Part model, mm, in its own coordinate system. A direction names the side the tool comes from. Give positions to 0.01 mm unless a question says otherwise; leave off trailing zeros. Loops run counter-clockwise (first coordinate to the right, second up) from the corner with the lowest first, then second, coordinate; pieces in that order, holes last. Notation, with made-up numbers: M 58.5,80 L 100.5,80 A31 cw 100.5,108 Z; hole C -36.5,37.25 d9. An arc over 180 degrees is marked long. Answer in a Markdown table with one row per item.
from build123d import *

# Parameters (mm, degrees)
SKETCH1_W                       = 101.6
SKETCH1_H                       = 59.436
BASE_EXTRUDE_DEPTH              = 3.81
BASE_CORNER_FILLET_R            = 2.54
SKETCH3_W                       = 3.81
SKETCH3_H                       = 3.81
PEG_EXTRUDE_DEPTH               = 2.54
MATERIAL_REMOVAL_CUT_DEPTH      = 120.96788652
SKETCH5_R                       = 1.905
REMOTE_CONTROL_HOLDER_CUT_DEPTH = 120.96788652


with BuildPart() as part:
    # Sketch1 → Base Extrude (new body)
    with BuildSketch(Plane(origin=(0, 0, 0), x_dir=(1, 0, 0), z_dir=(0, 1, 0))):
        with Locations((50.8, 29.718)):
            Rectangle(SKETCH1_W, SKETCH1_H)
    extrude(amount=BASE_EXTRUDE_DEPTH)

    # Base Corner Fillet
    base_corner_fillet_edges = [part.edges().sort_by_distance(p)[0] for p in [
        (0, 1.905, -59.436),
        (101.6, 1.905, -59.436),
        (101.6, 1.905, 0),
        (0, 1.905, 0),
    ]]
    fillet(base_corner_fillet_edges, radius=BASE_CORNER_FILLET_R)

    # Sketch3 → Peg Extrude (add)
    with BuildSketch(Plane.ZY):
        with Locations((-20.193, 1.905)):
            Rectangle(SKETCH3_W, SKETCH3_H)
        with Locations((-39.243, 1.905)):
            Rectangle(SKETCH3_W, SKETCH3_H)
    peg_extrude = extrude(amount=PEG_EXTRUDE_DEPTH)

    # Peg Mirror: Peg Extrude across plane
    add(peg_extrude.mirror(Plane(origin=(50.8, 0, 0), x_dir=(0, 0, 1), z_dir=(1, 0, 0))))

    # Sketch4 → Material Removal Cut (cut, through all)
    with BuildSketch(Plane.XZ):
        with BuildLine():
            Line((19.05, -12.7), (82.55, -12.7))
            ThreePointArc((82.55, -12.7), (87.040128061, -14.559871939), (88.9, -19.05))
            Line((88.9, -19.05), (88.9, -40.386))
            ThreePointArc((88.9, -40.386), (87.040128061, -44.876128061), (82.55, -46.736))
            Line((82.55, -46.736), (19.05, -46.736))
            ThreePointArc((19.05, -46.736), (14.559871939, -44.876128061), (12.7, -40.386))
            Line((12.7, -40.386), (12.7, -19.05))
            ThreePointArc((12.7, -19.05), (14.559871939, -14.559871939), (19.05, -12.7))
        make_face()
    extrude(amount=-MATERIAL_REMOVAL_CUT_DEPTH, mode=Mode.SUBTRACT)

    # Sketch5 → Remote Control Holder Cut (cut, through all)
    with BuildSketch(Plane(origin=(0, 3.81, 0), x_dir=(1, 0, 0), z_dir=(0, 1, 0))):
        with Locations(Location((63.5, 4.318, 0), (0, 0, 270))):
            Circle(SKETCH5_R)
        with Locations(Location((63.5, 55.118, 0), (0, 0, 270))):
            Circle(SKETCH5_R)
    extrude(amount=-REMOTE_CONTROL_HOLDER_CUT_DEPTH, mode=Mode.SUBTRACT)


solid = part.part
(1) Saw through at A-A (z = -32). Write the cut outline in (x, y), plus the area to 3 significant figures.
Recorded:
| item | result |
|---|---|
| outline | M 0,0 L 12.7,0 L 12.7,3.81 L 0,3.81 Z; M 88.9,0 L 101.6,0 L 101.6,3.81 L 88.9,3.81 Z |
| area | 96.8 mm^2 |
(2) Pin check, flat tips, straight feed: pin 1 Ø0.8 at (x, y) = (-1.5, 1) entering from +Z; pin 2 Ø1.9 at (y, z) = (2.5, -34.5) entering from -X; pin 3 Ø1.9 at (y, z) = (2.5, -28.5) entering from +X. Stop position of each tip, or through.
Recorded:
| item | result |
|---|---|
| pin 1 | stops at z = -18.29 |
| pin 2 | stops at x = 0 |
| pin 3 | stops at x = 101.6 |
(3) Which spindle directions (+Z, -Z, +X, -X, +Y, -Y) get a long thin tool onto all of the face, cutting with end or side? Do faces 1 (the face through (-1, 2, -18.288)), 2 (the face through (0, 2, -49)), 3 (the face through (101.6, 2, -49)), 4 (the face through (101.6, 2, -30)), 5 (the face through (50, 2, -12.7)). Say none if no direction does.
Recorded:
| item | result |
|---|---|
| face 1 | +Z, -X, +Y, -Y |
| face 2 | -Z, -X, +Y, -Y |
| face 3 | -Z, +X, +Y, -Y |
| face 4 | +X, +Y, -Y |
| face 5 | +Y, -Y |
(4) Pull direction Z, two halves, no side cores. Call faces 6 (the face through (87.089, 1.878, -44.826)), 7 (the face through (100.88, 1.93, -58.67)), 8 (the face through (103, 2, -37.338)), 9 (the face through (0, 2, -10)): +Z half, -Z half, draft (parallel to the pull), parting line (faces both ways), or undercut.
Recorded:
| item | result |
|---|---|
| face 6 | undercut |
| face 7 | -Z half |
| face 8 | undercut |
| face 9 | draft |
(5) Drill centre lines: line 1 along X through (y, z) = (0.9, -38.5); line 2 along X through (y, z) = (3.2, -37); line 3 along Z through (x, y) = (36, 1.45). Where is each one in solid material? Low to high.
Recorded:
| item | result |
|---|---|
| line 1 | x = -2.54 to 12.7, 88.9 to 104.14 |
| line 2 | x = 0 to 12.7, 88.9 to 101.6 |
| line 3 | z = -59.44 to -46.74, -12.7 to 0 |
(6) Saw through at C-C (y = 2.05). Give the number of separate pieces and of enclosed holes in the cut face, plus the area to 3 significant figures.
Recorded:
| item | result |
|---|---|
| separate pieces | 1 |
| enclosed holes | 3 |
| area | 3,490 mm^2 |
(7) Saw through at B-B (x = 63.5). Write the cut outline in (y, z).
Recorded:
| item | result |
|---|---|
| outline | M 0,-59.44 L 3.81,-59.44 L 3.81,-57.02 L 0,-57.02 Z; M 0,-53.21 L 3.81,-53.21 L 3.81,-46.74 L 0,-46.74 Z; M 0,-12.7 L 3.81,-12.7 L 3.81,-6.22 L 0,-6.22 Z; M 0,-2.41 L 3.81,-2.41 L 3.81,0 L 0,0 Z |
(8) Saw through at D-D (x = 86.5). Write the cut outline in (y, z).
Recorded:
| item | result |
|---|---|
| outline | M 0,-59.44 L 3.81,-59.44 L 3.81,-45.36 L 0,-45.36 Z; M 0,-14.08 L 3.81,-14.08 L 3.81,0 L 0,0 Z |
